For this review, take the finished solid that the model builds, in its own axes (mm). Give positions to 0.01 mm unless a question says otherwise; leave off trailing zeros. Write each loop counter-clockwise with the first axis right and the second up, starting at its lowest first coordinate (ties: lowest second). Pieces come first, ordered by that corner, then holes. Notation, with made-up numbers: M 26,78 L 40,78 A20 ccw 40,107 Z; hole C 5.25,-11.5 d4. An arc over 180 degrees is marked long. One line per item, written item: value. Start each with the question number.
Item 1: To check wall thickness, follow probe 1 along Z at (x, y) = (-48, -3); probe 2 along Z at (x, y) = (381.5, -17); probe 3 along X at (y, z) = (-3, 30.5). State the ranges of each line that lie inside material, in increasing order.
Item 2: Consider section A-A, the plane y = -6. Write out the cut boundary in (x, z).
Item 3: Consider section B-B, the plane z = 120. Write out the cut boundary in (x, y).
Item 4: Clearance check with flat-ended pins moving along their axes: pin 1 Ø1 at (y, z) = (-5.5, 231) entering from +X; pin 2 Ø1.5 at (y, z) = (-4.5, -12) entering from -X; pin 3 Ø4 at (x, y) = (341, -11) entering from +Z; pin 4 Ø4 at (x, z) = (127.5, 225.5) entering from +Y. State where each tip first meets the part, or that it passes through.
Item 5: Consider section C-C, the plane x = 385. Write out the cut boundary in (y, z).
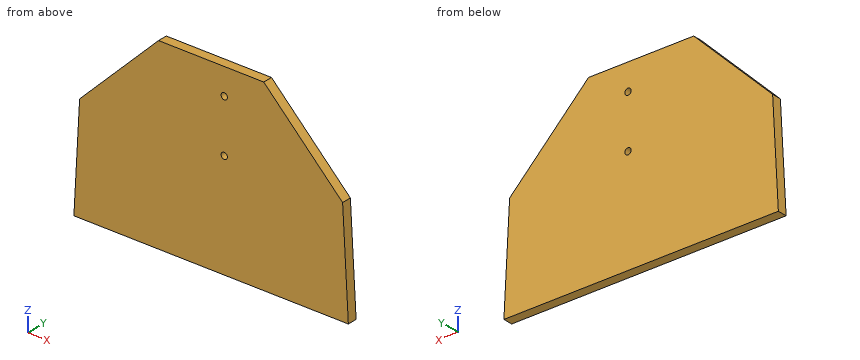
```python
from build123d import *

# Parameters (mm, degrees)
F1_DEPTH = 18
F3_R     = 6
F4_DEPTH = 25


with BuildPart() as f1:
    # F0 (on Front) → F1 (new body)
    with BuildSketch(Plane.XZ):
        Polygon((180.357315, 283.020994), (180.357315, -66.979006), (441.269071, -66.979006), (430.357315, 133.020994), (280.357315, 283.020994), align=None)
    extrude(amount=F1_DEPTH)

    # F2: F1 across face


with BuildPart() as f1_1:
    add(f1.part)
    add(f1.part.mirror(Plane(origin=(180.357315, -9, 108.020994), x_dir=(0, -1, 0), z_dir=(-1, 0, 0))))

    # F3 (on face) → F4 (cut)
    with BuildSketch(Plane.XZ.offset(18)):
        with Locations((205.357315, 233.020994)):
            Circle(F3_R)
        with Locations((205.357315, 133.020994)):
            Circle(F3_R)
    extrude(amount=-F4_DEPTH, mode=Mode.SUBTRACT)


solid = f1_1.part
```
Model answer:
1. probe 1: z = -66.98 to 154.66
1. probe 2: z = -66.98 to 181.88
1. probe 3: x = -75.24 to 435.95
2. outline: M -80.55,-66.98 L 441.27,-66.98 L 430.36,133.02 L 280.36,283.02 L 80.36,283.02 L -69.64,133.02 Z; hole C 205.36,133.02 d12; hole C 205.36,233.02 d12
3. outline: M -70.35,-18 L 431.07,-18 L 431.07,0 L -70.35,0 Z
4. pin 1: stops at x = 332.88
4. pin 2: stops at x = -77.6
4. pin 3: stops at z = 224.38
4. pin 4: stops at y = 0
5. outline: M -18,-66.98 L 0,-66.98 L 0,178.38 L -18,178.38 Z
